Read the model definition and answer for the solid it produces. Units are mm, in the model's axes. A direction names the side the tool comes from. Round coordinates to 2 decimals unless told otherwise and drop trailing zeros. Order: outer loops, then holes, each group sorted by start corner. A loop starts at its lowest first (then second) coordinate and runs counter-clockwise, first axis right, second up.
from build123d import *

# Parameters (mm, degrees)
ESBO_O1_W                  = 170
ESBO_O1_H                  = 30
RESSALTO_EXTRUS_O1_DEPTH   = 150
CORTE_EXTRUS_O1_DEPTH      = 222
CORTE_EXTRUS_O1_DEPTH_BACK = 36
RESSALTO_EXTRUS_O2_DEPTH   = 5
RESSALTO_EXTRUS_O3_DEPTH   = 5
ESBO_O4_W                  = 159.333333333
ESBO_O4_H                  = 140.588235294
CORTE_EXTRUS_O2_DEPTH      = 25
CORTE_EXTRUS_O3_DEPTH      = 31
CORTE_EXTRUS_O4_DEPTH      = 42
FILETE1_R                  = 10
CORTE_EXTRUS_O5_DEPTH      = 32
CORTE_EXTRUS_O6_START      = -15.72292277
CORTE_EXTRUS_O6_OUTLINE_R  = 3.95
CORTE_EXTRUS_O6_DEPTH      = 4.876648775
CORTE_EXTRUS_O7_START      = -132.751356438
CORTE_EXTRUS_O7_OUTLINE_R  = 3.95
CORTE_EXTRUS_O7_DEPTH      = 3.479370229
RESSALTO_EXTRUS_O6_DEPTH   = 17
RESSALTO_EXTRUS_O7_DEPTH   = 4
CORTE_EXTRUS_O8_DEPTH      = 21
F_3DSKETCH12_R             = 1.5
CORTE_EXTRUS_O9_DEPTH      = 14
CORTE_EXTRUS_O10_DEPTH     = 19
ESBO_O11_W                 = 17.407525744
ESBO_O11_H                 = 16.792397695
CORTE_EXTRUS_O11_DEPTH     = 10
CORTE_EXTRUS_O12_DEPTH     = 20
CORTE_EXTRUS_O13_DEPTH     = 14
CORTE_EXTRUS_O14_DEPTH     = 131


# Read off the part's stored shape, not the designer's step: Corte-extrusão6, Corte-extrusão7
with BuildPart() as part:
    # Esboço1 → Ressalto-extrusão1 (new body)
    with BuildSketch(Plane(origin=(0, 0, 0), x_dir=(1, 0, 0), z_dir=(0, 1, 0))):
        with Locations((85, 15)):
            Rectangle(ESBO_O1_W, ESBO_O1_H)
        Polygon((80, 160), (0, 30), (170, 30), (170, 160), align=None)
        Polygon((170, 160), (170, 185), (80, 160), align=None)
    extrude(amount=RESSALTO_EXTRUS_O1_DEPTH)

    # Esboço2 → Corte-extrusão1 (cut, two sides: drawn at the far end of the back side and taken through both)
    with BuildSketch(Plane(origin=(0, 0, 0), x_dir=(1, 0, 0), z_dir=(0, 1, 0)).offset(-CORTE_EXTRUS_O1_DEPTH_BACK)):
        Polygon((84.391050739, 157.608625205), (165, 180), (165, 5), (5, 5), (5, 29.866892941), align=None)
    extrude(amount=CORTE_EXTRUS_O1_DEPTH + CORTE_EXTRUS_O1_DEPTH_BACK, mode=Mode.SUBTRACT)

    # Esboço3 → Ressalto-extrusão2 (add)
    with BuildSketch(Plane(origin=(0, 0, 0), x_dir=(1, 0, 0), z_dir=(0, 1, 0))):
        Polygon((84.391050739, 157.608625205), (165, 180), (165, 5), (5, 5), (5, 29.866892941), align=None)
    extrude(amount=RESSALTO_EXTRUS_O2_DEPTH)

    # 3DSketch2 → Ressalto-extrusão3 (add)
    with BuildSketch(Plane(origin=(165, 150, -5), x_dir=(0, 0, -1), z_dir=(0, 1, 0))):
        Polygon((0, 0), (0, 160), (24.866892941, 160), (152.608625205, 80.608949261), (175, 0), align=None)
    extrude(amount=-RESSALTO_EXTRUS_O3_DEPTH)

    # Esboço4 → Corte-extrusão2 (cut)
    with BuildSketch(Plane.XY):
        with Locations((85.333333333, 74.705882353)):
            Rectangle(ESBO_O4_W, ESBO_O4_H)
    extrude(amount=-CORTE_EXTRUS_O2_DEPTH, mode=Mode.SUBTRACT)

    # 3DSketch3 → Corte-extrusão3 (cut)
    with BuildSketch(Plane(origin=(74.759025743, 90, -151.483416833), x_dir=(-0.29071694485714406, -0.8320502943378435, 0.4724150353928592), z_dir=(-0.8516583167045438, 0, -0.5240974256643346))):
        Polygon((0, 0), (22.188007849, 33.282011774), (72.111025509, 0), (49.92301766, -33.282011774), align=None)
    extrude(amount=-CORTE_EXTRUS_O3_DEPTH, mode=Mode.SUBTRACT)

    # 3DSketch4 → Corte-extrusão4 (cut)
    with BuildSketch(Plane(origin=(69.518051487, 130, -142.966833666), x_dir=(-0.37059284368967266, -0.7071067811865471, 0.6022133709956982), z_dir=(0.8516583167045362, 0, 0.5240974256643472))):
        Polygon((0, 0), (14.142135624, -14.142135624), (28.284271247, 0), (14.142135624, 14.142135624), align=None)
    extrude(amount=CORTE_EXTRUS_O4_DEPTH, mode=Mode.SUBTRACT)

    # Filete1
    filete1_edges = [part.edges().sort_by_distance(p)[0] for p in [
        (170, 75, -185),
        (125, 0, -172.5),
        (125, 150, -172.5),
        (80, 75, -160),
        (40, 0, -95),
        (40, 150, -95),
        (0, 75, -30),
        (84.391050739, 75, -157.608625205),
    ]]
    fillet(filete1_edges, radius=FILETE1_R)

    # 3DSketch5 → Corte-extrusão5 (cut)
    with BuildSketch(Plane(origin=(38.121221288, 25, -91.946984593), x_dir=(-0.194644897392922, 0.9284766908852593, 0.31629795826349816), z_dir=(0.851658316704544, 0, 0.5240974256643347))):
        Polygon((0, 0), (14.855627054, 37.139067635), (107.703296143, 0), (92.847669089, -37.139067635), align=None)
    extrude(amount=CORTE_EXTRUS_O5_DEPTH, mode=Mode.SUBTRACT)

    # Corte-extrusão6 outline → Corte-extrusão6 (cut)
    with BuildSketch(Plane(origin=(0, 0, 0), x_dir=(0.5240974256643349, 0, -0.8516583167045437), z_dir=(0.8516583167045437, 0, 0.5240974256643349)).offset(CORTE_EXTRUS_O6_START)):
        with Locations((148.193124726, 20)):
            Circle(CORTE_EXTRUS_O6_OUTLINE_R)
    extrude(amount=CORTE_EXTRUS_O6_DEPTH, mode=Mode.SUBTRACT)

    # Corte-extrusão7 outline → Corte-extrusão7 (cut)
    with BuildSketch(Plane(origin=(0, 0, 0), x_dir=(0.9635179096299408, 0, -0.267643863786094), z_dir=(0.267643863786094, 0, 0.9635179096299409)).offset(CORTE_EXTRUS_O7_START)):
        with Locations((161.993020775, 122.164347625)):
            Circle(CORTE_EXTRUS_O7_OUTLINE_R)
    extrude(amount=CORTE_EXTRUS_O7_DEPTH, mode=Mode.SUBTRACT)

    # 3DSketch9 → Ressalto-extrusão6 (add)
    with BuildSketch(Plane(origin=(76.350750718, 26, -154.069969916), x_dir=(-0.29815073011621673, 0.8224176546598938, 0.4844949364388514), z_dir=(0.8516583167045438, 0, 0.5240974256643349))):
        Polygon((0, 0), (26.758649409, 38.684123705), (82.683049926, 0), (55.924400517, -38.684123705), align=None)
        Polygon((5.017416454, 0.222210211), (27.772783339, 33.118916398), (77.117842619, -1.01413393), (54.362475733, -33.910840117), align=None, mode=Mode.SUBTRACT)
    extrude(amount=RESSALTO_EXTRUS_O6_DEPTH)

    # 3DSketch10 → Ressalto-extrusão7 (add, along a direction that is not the sketch's normal)
    with BuildSketch(Plane(origin=(0, 0, 0), x_dir=(0.7498378553650926, 0.6616216370868463, 0), z_dir=(0, 0, 1))):
        with BuildLine():
            Line((0, 0), (14.996757107, -13.232432742))
            Line((14.996757107, -13.232432742), (28.229189849, 1.764324366))
            ThreePointArc((28.229189849, 1.764324366), (21.556867541, 14.536675999), (25.141622209, 28.493838504))
            Line((25.141622209, 28.493838504), (13.232432742, 14.996757107))
            Line((13.232432742, 14.996757107), (0, 0))
        make_face()
        with BuildLine():
            Line((99.243245563, 112.475678305), (115.742930564, 97.917132715))
            Line((115.742930564, 97.917132715), (100.070543679, 80.155094246))
            ThreePointArc((100.070543679, 80.155094246), (86.055529464, 85.755516688), (71.66166921, 81.216558438))
            Line((71.66166921, 81.216558438), (83.570858678, 94.713639835))
            Line((83.570858678, 94.713639835), (99.243245563, 112.475678305))
        make_face()
        Polygon((226.715680975, 0), (211.718923868, 13.232432742), (198.486491126, -1.764324366), (213.483248233, -14.996757107), align=None)
        Polygon((127.472435412, -112.475678305), (112.475678305, -99.243245563), (125.708111047, -84.246488456), (140.704868154, -97.478921197), align=None)
    extrude(amount=-RESSALTO_EXTRUS_O7_DEPTH, dir=(0.26764386378609445, 0, 0.9635179096299407))

    # 3DSketch11 → Corte-extrusão8 (cut)
    with BuildSketch(Plane(origin=(153.100052242, 17.26943239, -180.305570067), x_dir=(-0.07376023038027929, 0.9970655099962036, 0.02048895288341091), z_dir=(0.2676438637860946, 0, 0.9635179096299407))):
        Polygon((0, 0), (0.269964353, 3.516152018), (46.066103253, 0), (45.7961389, -3.516152018), align=None)
    extrude(amount=CORTE_EXTRUS_O8_DEPTH, mode=Mode.SUBTRACT)

    # 3DSketch12 → Corte-extrusão9 (cut)
    with BuildSketch(Plane(origin=(160, 140, 0), x_dir=(-0.7560654573770964, -0.6544960077503622, 0), z_dir=(0, 0, 1))):
        with Locations(Location((0, 0, 0), (0, 0, 319.118554366))):
            Circle(F_3DSKETCH12_R)
        with Locations(Location((85.084481008, 98.288509459, 0), (0, 0, 319.118554366))):
            Circle(F_3DSKETCH12_R)
        with Locations(Location((113.858951537, -96.124361942, 0), (0, 0, 139.118554366))):
            Circle(F_3DSKETCH12_R)
        with Locations(Location((196.909602971, 0, 0), (0, 0, 139.118554366))):
            Circle(F_3DSKETCH12_R)
    extrude(amount=-CORTE_EXTRUS_O9_DEPTH, mode=Mode.SUBTRACT)

    # 3DSketch13 → Corte-extrusão10 (cut)
    with BuildSketch(Plane(origin=(170, 70.245878967, 0), x_dir=(0, -0.4354246522459521, -0.9002251786172678), z_dir=(-1, 0, 0))):
        Polygon((0, 0), (32.261446294, -15.604350297), (39.809023237, 0), (7.547576943, 15.604350297), align=None)
    extrude(amount=CORTE_EXTRUS_O10_DEPTH, mode=Mode.SUBTRACT)

    # Esboço11 → Corte-extrusão11 (cut)
    with BuildSketch(Plane(origin=(170, 0, 0), x_dir=(0, 0, -1), z_dir=(1, 0, 0))):
        with Locations((8.703762872, 30.096304842)):
            Rectangle(ESBO_O11_W, ESBO_O11_H)
    extrude(amount=-CORTE_EXTRUS_O11_DEPTH, mode=Mode.SUBTRACT)

    # 3DSketch14 → Corte-extrusão12 (cut)
    with BuildSketch(Plane(origin=(170, 87.396079578, 0), x_dir=(0, -0.09341146144778735, -0.9956275904524686), z_dir=(1, 0, 0))):
        Polygon((0, 0), (20.627912038, 1.935345533), (19.506160301, 13.891554783), (-1.121751737, 11.956209249), align=None)
        Polygon((-2.576084268, 27.457236328), (18.165947056, 29.403288726), (16.691971594, 45.113680317), (-4.050059731, 43.167627919), align=None)
        Polygon((91.534016736, 10.656116635), (99.096194716, 11.679615344), (100.676965661, 0), (93.114787682, -1.02349871), align=None)
    extrude(amount=-CORTE_EXTRUS_O12_DEPTH, mode=Mode.SUBTRACT)

    # 3DSketch15 → Corte-extrusão13 (cut)
    with BuildSketch(Plane(origin=(129.748977416, 150, 0), x_dir=(-0.6170578351280018, 0, -0.7869178026370631), z_dir=(0, -1, 0))):
        Polygon((0, 0), (11.819817446, 9.268453377), (19.087630878, 0), (7.267813432, -9.268453377), align=None)
    extrude(amount=CORTE_EXTRUS_O13_DEPTH, mode=Mode.SUBTRACT)

    # 3DSketch16 → Corte-extrusão14 (cut, along a direction that is not the sketch's normal)
    with BuildSketch(Plane(origin=(-4.487914591, 154.677224746, -90), x_dir=(0.7478301848964537, -0.6638900621019538, 0), z_dir=(0, 0, 1))):
        Polygon((0, 0), (133.725190167, 118.715219842), (239.115232272, 0), (105.390042105, -118.715219842), align=None)
    extrude(amount=-CORTE_EXTRUS_O14_DEPTH, dir=(-0.5240974256643347, 0, 0.8516583167045438), mode=Mode.SUBTRACT)


solid = part.part
Q1. Flat-ended cylindrical pins translate along their axes: pin 1 (7.5 mm diameter, centred on x = 153, y = 140, fed in from -Z); pin 2 (2.5 mm diameter, centred on x = 11, y = 138.16, fed in from +Z); pin 3 (6 mm diameter, centred on y = 59.5, z = -46, fed in from -X). Find the tip coordinate at first contact, or state that the pin passes through.
Outcome:
pin 1: stops at z = -3.85
pin 2: stops at z = -37.51
pin 3: stops at x = 8
Q2. For a pull along Y with two mould halves and no side action, classify faces 1 (the face through (21.477, 135.787, -1.9)), 2 (the face through (168, 70.246, -18)), 3 (the face through (0.37, 75.98, -29.86)) as released by +Y, released by -Y, zero draft, split by the parting line, or undercut.
Outcome:
face 1: undercut
face 2: undercut
face 3: zero draft
Q3. A cutting plane is placed at C-C, the plane y = 81. Give the vertices of the cut face in (x, z), plus the area to 3 significant figures.
Outcome:
outline: (0, -27.17) arc R10 ccw to (1.48, -32.41) - (17.16, -57.88) - (20.96, -55.54) - (5, -29.87) - (5, -5) - (5.67, -5) - (5.67, 0) - (0, 0) - close; (41.29, -90) - (42.37, -90) - (42.07, -89.52) - close; (165, -90) - (170, -90) - (170, 0) - (165, 0) - close
area: 741 mm2
Q4. For faces 4 (the face through (169, 79, -90)), 5 (the face through (12, 135, -3.854)), 6 (the face through (129.749, 148, -7)), 7 (the face through (167, 79, 0)), 8 (the face through (168, 52.912, -18)), determine the directions among +Z, -Z, +X, -X, +Y, -Y from which every point of the face is accessible in a straight line to the end or side of a thin tool.
Outcome:
face 4: -Z, +X, -X, +Y, -Y
face 5: none
face 6: +Z, +Y
face 7: +Z, +X, -X, +Y, -Y
face 8: +Z, +X
Q5. Straight lines are drawn through the part: probe 1 along Y at (x, z) = (160, -1.5); probe 2 along Y at (x, z) = (90, -36.5); probe 3 along X at (y, z) = (21.5, -16.5). For each, find the intervals that lie inside material, in ascending order.
Outcome:
probe 1: y = 0 to 8.5, 11.5 to 20, 130.75 to 138.5, 141.5 to 150
probe 2: y = 0 to 5, 145 to 150
probe 3: x = 0 to 5, 165 to 170
Q6. A cutting plane is placed at B-B, the plane x = 59. Give the vertices of the cut face in (y, z), plus the area to 3 significant figures.
Outcome:
outline: (0, -90) - (5, -90) - (5, -25) - (4.41, -25) - (4.41, 0) - (0, 0) - close; (145, -90) - (150, -90) - (150, 0) - (145, 0) - close
area: 885 mm2
Q7. A cutting plane is placed at A-A, the plane y = 56. Give the vertices of the cut face in (x, z), plus the area to 3 significant figures.
Outcome:
outline: (0, -27.17) arc R10 ccw to (1.48, -32.41) - (17.16, -57.88) - (20.96, -55.54) - (5, -29.87) - (5, -5) - (5.67, -5) - (5.67, 0) - (0, 0) - close; (41.29, -90) - (42.37, -90) - (42.07, -89.52) - close; (165, -90) - (170, -90) - (170, -35.84) - (165, -35.84) - close
area: 562 mm2
